Geometry: final body of the model. Coordinates: model frame, mm. Face numbers are marked on the shaded views. A direction names the side the tool comes from. Round coordinates to 2 decimals unless told otherwise and drop trailing zeros. Loops run counter-clockwise (first coordinate to the right, second up) from the corner with the lowest first, then second, coordinate; pieces in that order, holes last. Notation, with made-up numbers: M 52.5,19 L 58.5,19 A24 cw 58.5,54 Z; hole C -20.5,-21 d7. An arc over 180 degrees is marked long. Answer as a JSON object with one key per item and string values.
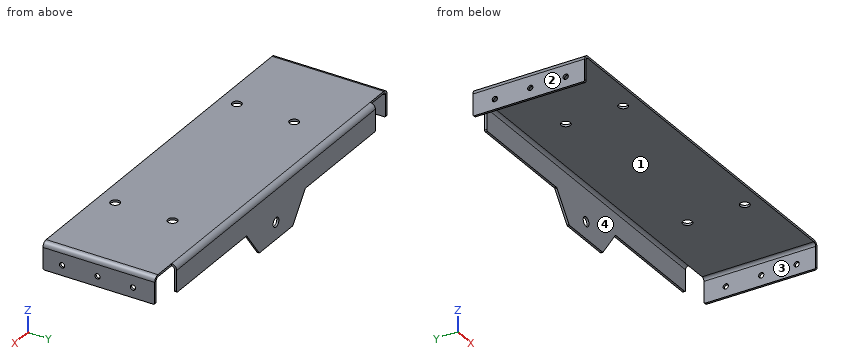
```python
from build123d import *

# Parameters (mm, degrees)
SKETCH1_W                                 = 351.6122
SKETCH1_H                                 = 105.156
BASE_FLANGE1_DEPTH                        = 1.9939
EDGE_FLANGE1_STRIP_W                      = 13.66774
EDGE_FLANGE1_STRIP_H                      = 1.9939
EDGE_FLANGE1_STRIP_CUT_DEPTH              = 105.156
EDGE_FLANGE1_STRIP_2_W                    = 13.66774
EDGE_FLANGE1_STRIP_2_H                    = 1.9939
EDGE_FLANGE1_STRIP_CUT_2_DEPTH            = 105.156
EDGE_FLANGE1_DEPTH                        = 105.156
EDGE_FLANGE1_BEND_DEPTH                   = 105.156
EDGE_FLANGE2_DEPTH                        = 300.8122
EDGE_FLANGE2_START                        = 1.9939
EDGE_FLANGE2_FLAT_DEPTH                   = 1.9939
F_0_221_DIAMETER_HOLE1_D                  = 4.9149
HOLE_FOR_1_4_SELF_CLINCHING_NUTS_S_SS_C_D = 8.7376
HOLE_FOR_1_4_SELF_CLINCHING_NUTS_S_2_D    = 8.7376
FILLET1_R                                 = 1.27


# Sheet-metal steps are written as plain solids
with BuildPart() as part:
    # Sketch1 → Base-Flange1 (new body)
    with BuildSketch(Plane.XY):
        with Locations((175.8061, 52.578)):
            Rectangle(SKETCH1_W, SKETCH1_H)
    extrude(amount=-BASE_FLANGE1_DEPTH)

    # Edge-Flange1 strip (across the edge) → Edge-Flange1 strip cut (cut)
    with BuildSketch(Plane(origin=(0, 0, -1.9939), x_dir=(1, 0, 0), z_dir=(0, 1, 0))):
        with Locations((-1.9939, -0.99695)):
            Rectangle(EDGE_FLANGE1_STRIP_W, EDGE_FLANGE1_STRIP_H)
    extrude(amount=EDGE_FLANGE1_STRIP_CUT_DEPTH, mode=Mode.SUBTRACT)

    # Edge-Flange1 strip 2 (across the edge) → Edge-Flange1 strip cut 2 (cut)
    with BuildSketch(Plane(origin=(351.6122, 105.156, -1.9939), x_dir=(-1, 0, 0), z_dir=(0, -1, 0))):
        with Locations((-1.9939, -0.99695)):
            Rectangle(EDGE_FLANGE1_STRIP_2_W, EDGE_FLANGE1_STRIP_2_H)
    extrude(amount=EDGE_FLANGE1_STRIP_CUT_2_DEPTH, mode=Mode.SUBTRACT)

    # Edge-Flange1 section (across the edge) → Edge-Flange1 (add)
    with BuildSketch(Plane(origin=(0, 0, -1.9939), x_dir=(1, 0, 0), z_dir=(0, 1, 0))):
        with BuildLine():
            Line((0, 2.84607), (0, 23.4061))
            Line((0, 23.4061), (1.9939, 23.4061))
            Line((1.9939, 23.4061), (1.9939, 2.84607))
            ThreePointArc((1.9939, 2.84607), (2.827494603, 0.833594603), (4.83997, 0))
            Line((4.83997, 0), (4.83997, -1.9939))
            ThreePointArc((4.83997, -1.9939), (1.417594392, -0.576305608), (0, 2.84607))
        make_face()
    extrude(amount=EDGE_FLANGE1_DEPTH)

    # Edge-Flange1 section 2 (across the edge) → Edge-Flange1 bend (add)
    with BuildSketch(Plane(origin=(351.6122, 105.156, -1.9939), x_dir=(-1, 0, 0), z_dir=(0, -1, 0))):
        with BuildLine():
            Line((0, 2.84607), (0, 23.4061))
            Line((0, 23.4061), (1.9939, 23.4061))
            Line((1.9939, 23.4061), (1.9939, 2.84607))
            ThreePointArc((1.9939, 2.84607), (2.827494603, 0.833594603), (4.83997, 0))
            Line((4.83997, 0), (4.83997, -1.9939))
            ThreePointArc((4.83997, -1.9939), (1.417594392, -0.576305608), (0, 2.84607))
        make_face()
    extrude(amount=EDGE_FLANGE1_BEND_DEPTH)

    # Edge-Flange2 bend section (across the edge) → Edge-Flange2 (add)
    with BuildSketch(Plane(origin=(25.4, 108.00207, -1.9939), x_dir=(0, -1, 0), z_dir=(1, 0, 0))):
        with BuildLine():
            Line((-1.9939, 2.84607), (0, 2.84607))
            ThreePointArc((0, 2.84607), (0.833594603, 0.833594603), (2.84607, 0))
            Line((2.84607, 0), (2.84607, -1.9939))
            ThreePointArc((2.84607, -1.9939), (-0.576305608, -0.576305608), (-1.9939, 2.84607))
        make_face()
    extrude(amount=EDGE_FLANGE2_DEPTH)

    # Edge-Flange2 profile (on flange) → Edge-Flange2 flat (add)
    with BuildSketch(Plane(origin=(0, 108.00207, -1.9939), x_dir=(1, 0, 0), z_dir=(0, 1, 0)).offset(EDGE_FLANGE2_START)):
        Polygon((326.2122, 2.84607), (326.2122, 23.4061), (220.2561, 23.4061), (201.2061, 48.8061), (150.4061, 48.8061), (131.3561, 23.4061), (25.4, 23.4061), (25.4, 2.84607), align=None)
    extrude(amount=-EDGE_FLANGE2_FLAT_DEPTH)

    # 0.221_ Diameter Hole1 (through all)
    with Locations(Plane(origin=(351.6122, 0, 0), x_dir=(0, 0, -1), z_dir=(1, 0, 0))):
        with Locations((15.875, 84.59597), (15.875, 17.92097), (15.875, 51.25847)):
            Hole(F_0_221_DIAMETER_HOLE1_D / 2)

    # Hole for 1_4 Self-clinching Nuts _S_SS_C (through all)
    with Locations(Plane(origin=(0, 109.99597, 0), x_dir=(1, 0, 0), z_dir=(0, 1, 0))):
        with Locations((175.8061, 34.925)):
            Hole(HOLE_FOR_1_4_SELF_CLINCHING_NUTS_S_SS_C_D / 2)

    # Hole for 1_4 Self-clinching Nuts _S_ 2 (through all)
    with Locations(Plane.XY):
        with Locations((83.7311, 69.86397), (83.7311, 15.88897), (267.8811, 15.88897), (267.8811, 69.86397)):
            Hole(HOLE_FOR_1_4_SELF_CLINCHING_NUTS_S_2_D / 2)

    # Fillet1
    fillet1_edges = [part.edges().sort_by_distance(p)[0] for p in [
        (0.99695, 0, -25.4),
        (0.99695, 105.156, -25.4),
        (350.61525, 105.156, -25.4),
        (350.61525, 0, -25.4),
        (25.4, 108.99902, -25.4),
        (326.2122, 108.99902, -25.4),
        (220.2561, 108.99902, -25.4),
        (201.2061, 108.99902, -50.8),
        (150.4061, 108.99902, -50.8),
        (131.3561, 108.99902, -25.4),
    ]]
    fillet(fillet1_edges, radius=FILLET1_R)


solid = part.part
```
1) Cut plane B-B on y = 60. Return the cut outline in (x, z), and give its area (3 significant figures).
Geometry results:
{"outline": "M 0,-25.4 L 1.99,-25.4 L 1.99,-4.84 A2.85 cw 4.84,-1.99 L 346.77,-1.99 A2.85 cw 349.62,-4.84 L 349.62,-25.4 L 351.61,-25.4 L 351.61,-4.84 A4.84 ccw 346.77,0 L 4.84,0 A4.84 ccw 0,-4.84 Z", "area": "788 mm2"}
2) Cut plane C-C on x = 254. Return the cut outline in (y, z), and give its area (3 significant figures).
Geometry results:
{"outline": "M 0,-1.99 L 105.16,-1.99 A2.85 cw 108,-4.84 L 108,-25.4 L 110,-25.4 L 110,-4.84 A4.84 ccw 105.16,0 L 0,0 Z", "area": "263 mm2"}
3) Cut plane A-A on x = 155. Return the cut outline in (y, z), and give its area (3 significant figures).
Geometry results:
{"outline": "M 0,-1.99 L 105.16,-1.99 A2.85 cw 108,-4.84 L 108,-50.8 L 110,-50.8 L 110,-4.84 A4.84 ccw 105.16,0 L 0,0 Z", "area": "313 mm2"}
4) Line query: probe 1 along X at (y, z) = (91, -10); probe 2 along Y at (x, z) = (265, -7.5); probe 3 along Z at (x, y) = (243.5, 88.5). Output: solid intervals per line, ascending.
Geometry results:
{"probe 1": "0 to 1.99, 349.62 to 351.61", "probe 2": "108 to 110", "probe 3": "-1.99 to 0"}
5) First-contact query: pin 1 (14 mm diameter, centred on x = 175.81, z = -34.92, fed in from -Y); pin 2 (6 mm diameter, centred on x = 299.5, y = 87, fed in from -Z); pin 3 (11.5 mm diameter, centred on x = 83.73, y = 69.86, fed in from +Z); pin 4 (0.6 mm diameter, centred on x = 1, y = 36, fed in from -Z). Flat tips, straight axial feed; report the tip coordinate or a pass-through.
Geometry results:
{"pin 1": "y = 108", "pin 2": "z = -1.99", "pin 3": "z = 0", "pin 4": "z = -25.4"}
6) Cut plane D-D on z = -44. Return the cut outline in (x, y).
Geometry results:
{"outline": "M 145.31,108 L 206.31,108 L 206.31,110 L 145.31,110 Z"}
7) Set-up query: the marked faces 1, 2, 3 and 4. Return all of +Z, -Z, +X, -X, +Y, -Y with unobstructed straight access to the full face (end or side cutting, diameter ignored); none if empty.
Geometry results:
{"face 1": "-Z, -Y", "face 2": "+Z, -Z, -X, +Y, -Y", "face 3": "-Z, +Y, -Y", "face 4": "-Z, +X, -X, -Y"}
